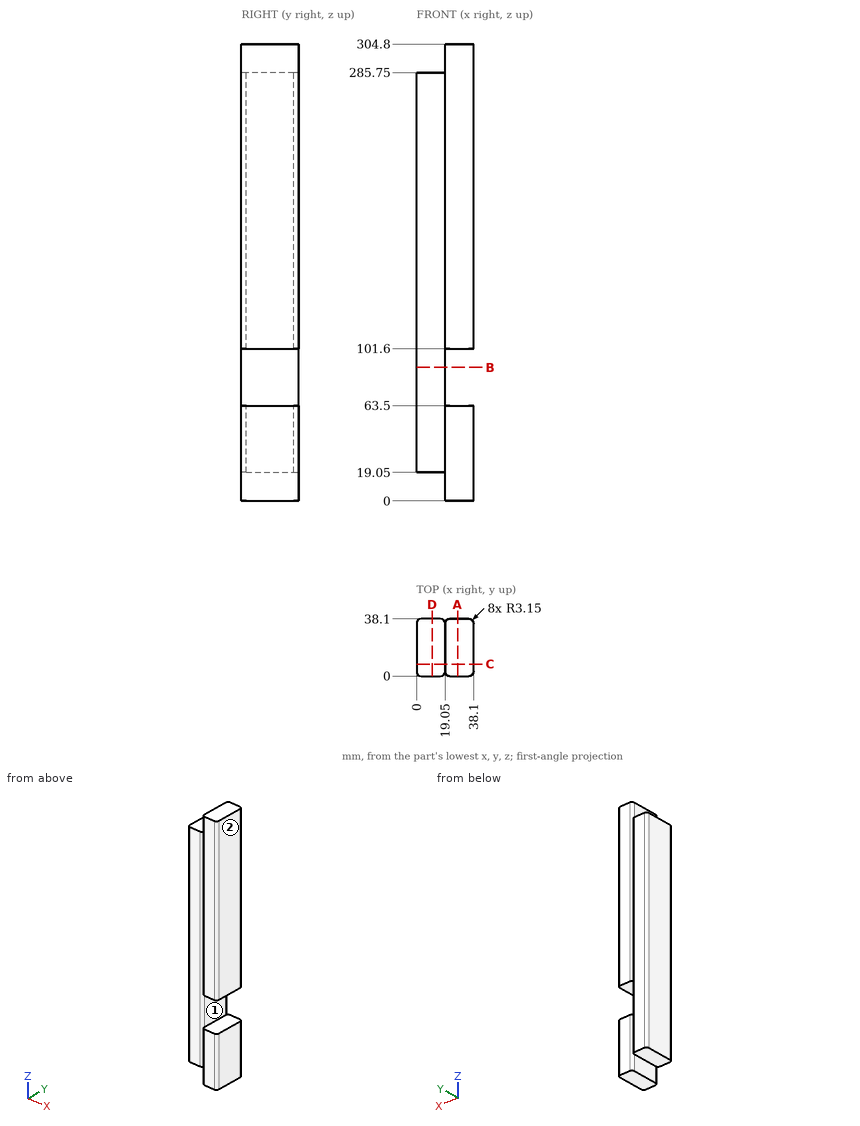
Drawing for the job (mm, zero at the part's lowest x, y, z). A direction names the side the tool comes from. Round coordinates to 2 decimals unless told otherwise and drop trailing zeros. Write each loop counter-clockwise with the first axis right and the second up, starting at its lowest first coordinate (ties: lowest second). Pieces come first, ordered by that corner, then holes. Notation, with made-up numbers: M 70,89 L 108,89 A29 ccw 108,113 Z; hole C 50.25,57 d3. An arc over 180 degrees is marked long. Put each result on its own line as item: value.
Item 1: Probe L1, parallel to Z at x = 36.5, y = 22.5; L2, parallel to Z at x = 11, y = 32; L3, parallel to Y at x = 3, z = 170.5. List the from-to ranges inside material, lowest first. Write a range as from..to.
Responses:
L1: 0..63.5, 101.6..304.8
L2: 19.05..285.75
L3: 0..38.1
Item 2: Cut at D-D (x = 10.5). List the corners of the cut face in (y, z), and give its area (3 significant figures).
Responses:
outline: M 0,19.05 L 38.1,19.05 L 38.1,285.75 L 0,285.75 Z
area: 10,200 mm²
Item 3: Cut at A-A (x = 27.5). List the corners of the cut face in (y, z), and give its area (3 significant figures).
Responses:
outline: M 0,0 L 38.1,0 L 38.1,63.5 L 0,63.5 Z; M 0,101.6 L 38.1,101.6 L 38.1,304.8 L 0,304.8 Z
area: 10,200 mm²
Item 4: Flat gauge pins, fed straight in: P1, Ø5.5, axis at y = 19, z = 5, coming from the -X side; P2, Ø1.5, axis at x = 5.5, y = 9, coming from the -Z side; P3, Ø15, axis at x = 7.5, y = 13, coming from the +Z side; P4, Ø5.5, axis at x = 24, y = 12, coming from the -Z side. Where does each tip first touch, or does it go through?
Responses:
P1: x = 19.05
P2: z = 19.05
P3: z = 285.75
P4: z = 0
Item 5: Cut at B-B (z = 89). List the corners of the cut face in (x, y), and give its area (3 significant figures).
Responses:
outline: M 0,3.15 A3.15 ccw 3.15,0 L 15.9,0 A3.15 ccw 19.05,3.15 L 19.05,34.95 A3.15 ccw 15.9,38.1 L 3.15,38.1 A3.15 ccw 0,34.95 Z
area: 717 mm²
Item 6: Tool access for the marked faces 1 and 2: list every direction of +Z, -Z, +X, -X, +Y, -Y with a clear straight run to the whole face (end or side of a thin tool).
Responses:
face 1: +X, +Y, -Y
face 2: +Z, -Z, +X, +Y, -Y
Item 7: Cut at C-C (y = 8). List the corners of the cut face in (x, z), and give its area (3 significant figures).
Responses:
outline: M 0,19.05 L 19.05,19.05 L 19.05,0 L 38.1,0 L 38.1,63.5 L 19.05,63.5 L 19.05,101.6 L 38.1,101.6 L 38.1,304.8 L 19.05,304.8 L 19.05,285.75 L 0,285.75 Z
area: 10,200 mm²
